Check sheet for the drawn part. Datum: minimum x, y, z corner. Units: mm. A direction names the side the tool comes from. Give positions to 0.01 mm unless a question says otherwise; leave off trailing zeros. Order: outer loops, then holes, each group sorted by start corner. A loop starts at its lowest first (then second) coordinate and runs counter-clockwise, first axis right, second up. Notation, with made-up numbers: M 67.25,-18 L 90.25,-18 A12 ccw 90.25,4 Z; hole C 62,10 d6. An arc over 180 degrees is marked long. One line per question, with ' | ' between items. Start each with the question number.
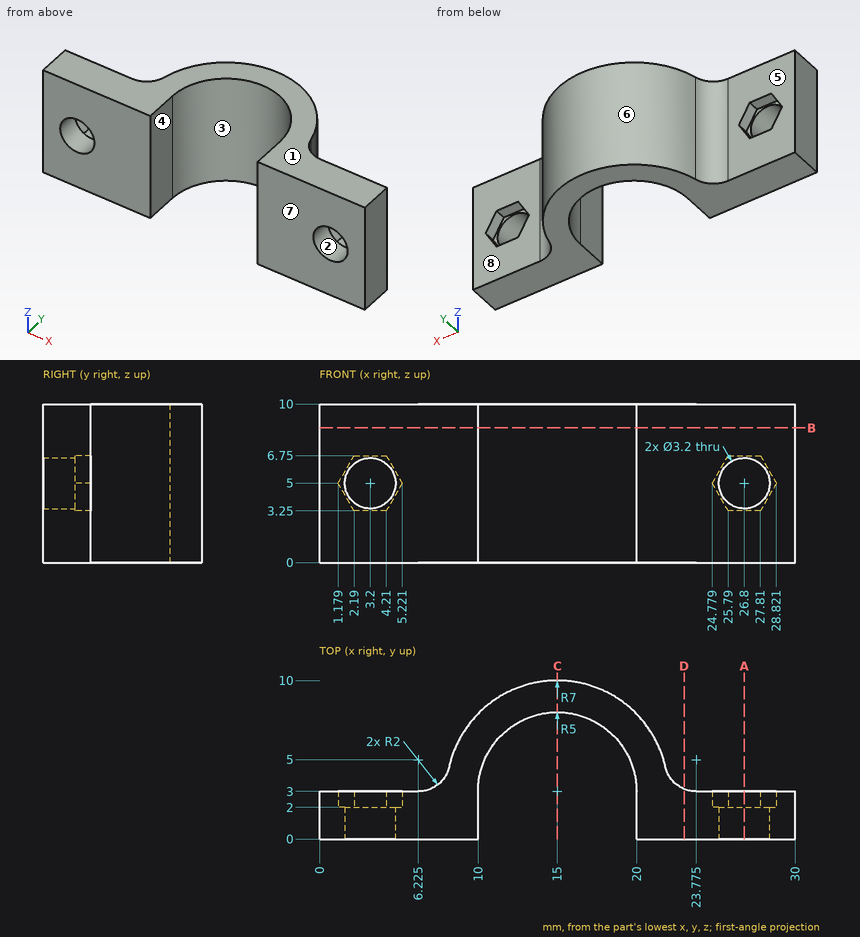
Item 1: Scan lines: probe 1 along Z at (x, y) = (26.8, 1.45); probe 2 along X at (y, z) = (1, 6); probe 3 along X at (y, z) = (1.25, 6.75). Record each from-to range of solid material in increasing order. Write a range as [from, to].
Item 2: Draft check along Z on the marked faces 1, 2 and 3. Enter one of: released by +Z, released by -Z, zero draft, split by the parting line, or undercut.
Item 3: Section check D-D, the plane x = 23. Record the cut outline in (y, z).
Item 4: Set-up check for the marked faces 4, 5, 6, 7 and 8: record each of +Z, -Z, +X, -X, +Y, -Y from which the full face is reachable in a straight line by a thin tool's end or side.
Item 5: Section check A-A, the plane x = 26.8. Record the cut outline in (y, z), then the cut area to 3 significant figures.
Item 6: Go/stop test with flat-tipped pins: P1, Ø5, axis at y = 7.5, z = 2, coming from the +X side; P2, Ø5, axis at x = 3.5, z = 4, coming from the +Y side; P3, Ø1, axis at x = 26, z = 6, coming from the +Y side. Record where each tip stops, or that it passes through.
Item 7: Section check B-B, the plane z = 8.5. Record the cut outline in (x, y) (1 decimal).
Item 8: Section check C-C, the plane x = 15. Record the cut outline in (y, z).
Reported:
1) probe 1: z = [0, 3.4], [6.6, 10] | probe 2: x = [0, 1.95], [4.45, 10], [20, 25.55], [28.05, 30] | probe 3: x = [0, 10], [20, 30]
2) face 1: released by +Z | face 2: undercut | face 3: zero draft
3) outline: M 0,0 L 3.16,0 L 3.16,10 L 0,10 Z
4) face 4: +Z, -Z, -Y | face 5: +Z, -Z, -X, +Y | face 6: +Z, -Z, +Y | face 7: +Z, -Z, +X, -X, -Y | face 8: +Z, -Z, +X, +Y
5) outline: M 0,0 L 3,0 L 3,3.25 L 2,3.25 L 2,3.4 L 0,3.4 Z; M 0,6.6 L 2,6.6 L 2,6.75 L 3,6.75 L 3,10 L 0,10 Z | area: 20.1 mm^2
6) P1: stops at x = 21.71 | P2: stops at y = 3 | P3: stops at y = 2
7) outline: M 0,0 L 10,0 L 10,3 A5 cw 20,3 L 20,0 L 30,0 L 30,3 L 23.8,3 A2 cw 21.8,4.6 A7 ccw 8.2,4.6 A2 cw 6.2,3 L 0,3 Z
8) outline: M 8,0 L 10,0 L 10,10 L 8,10 Z
